Work out the finished part from the listing and answer in its coordinate system (mm). A direction names the side the tool comes from. Round coordinates to 2 decimals unless told otherwise and drop trailing zeros. Loops run counter-clockwise (first coordinate to the right, second up) from the corner with the lowest first, then second, coordinate; pieces in that order, holes last. Notation, with made-up numbers: (-21.5, 60) - (28.5, 60) arc R23 cw to (28.5, 94) - close; hole circle Ø3 at (-6.5, 85.25). An arc over 180 degrees is marked (long way). Return JSON: item names as keys, results as strings.
from build123d import *

# Parameters (mm, degrees)
F1_W     = 10
F1_H     = 10
F2_DEPTH = 1
F3_W     = 10
F3_H     = 1
F4_DEPTH = 12
F8_W     = 1
F8_H     = 15
F10_R    = 3


with BuildPart() as f2:
    # F1 (on Top) → F2 (new body)
    with BuildSketch(Plane.XY):
        with Locations((-1.3497796124, 5)):
            Rectangle(F1_W, F1_H)
    extrude(amount=F2_DEPTH)

    # F3 (on face) → F4 (join)
    with BuildSketch(Plane.XY.offset(1)):
        with Locations((-1.3497796124, 9.5)):
            Rectangle(F3_W, F3_H)
    extrude(amount=F4_DEPTH)

    # F8 (on 3pt) → F9 (join, up to the next surface of F2)
    with BuildSketch(Plane(origin=(0, -0.48, 0.36), x_dir=(-1, 0, 0), z_dir=(0, 0.8, -0.6))):
        with Locations((1.3497796124, 8.3)):
            Rectangle(F8_W, F8_H)
    extrude(until=Until.NEXT)

    # F10
    f10_edges = [f2.edges().sort_by_distance(p)[0] for p in [
        (3.65022, 0, 0.5),
        (-6.34978, 0, 0.5),
    ]]
    fillet(f10_edges, radius=F10_R)


solid = f2.part
1) A tool of negligible diameter and unlimited length cuts with its end or side. For faces 1 (the flat face through (-6.35, 9.3, 5)), 2 (the flat face through (1, 5, 1)), 3 (the flat face through (-4, 5, 1)), from which of +Z, -Z, +X, -X, +Y, -Y can it reach the whole face along a straight path? Write none if from no direction.
Verdict:
{"face 1": "+Z, -Z, -X, +Y, -Y", "face 2": "+Z, +X, -Y", "face 3": "+Z, -X, -Y"}
2) Find the intervals of material crossed by L1, parallel to Z at x = -3.25, y = 7; L2, parallel to X at y = 6.25, z = 9; L3, parallel to Y at x = -2, z = 4, in increasing order.
Verdict:
{"L1": "z = 0 to 1", "L2": "x = -1.85 to -0.85", "L3": "y = 9 to 10"}
3) Section B-B (x = -1.5) is taken. Give the vertices of the cut face in (y, z).
Verdict:
{"outline": "(0, 0) - (10, 0) - (10, 13) - (9, 13) - (0, 1) - close"}
4) Section D-D (x = 0) is taken. Give the vertices of the cut face in (y, z), and give its area (3 significant figures).
Verdict:
{"outline": "(0, 0) - (10, 0) - (10, 13) - (9, 13) - (9, 1) - (0, 1) - close", "area": "22.0 mm2"}
5) Flat-ended cylindrical pins translate along their axes: pin 1 (1.3 mm diameter, centred on x = -4.5, z = 6, fed in from -Y); pin 2 (2.5 mm diameter, centred on x = 2, y = 3.5, fed in from +Z); pin 3 (2 mm diameter, centred on y = 2, z = 1.5, fed in from +X). Find the tip coordinate at first contact, or state that the pin passes through.
Verdict:
{"pin 1": "stops at y = 9", "pin 2": "stops at z = 1", "pin 3": "stops at x = 3.65"}
6) Section A-A (z = 9) is taken. Give the vertices of the cut face in (x, y), and give its area (3 significant figures).
Verdict:
{"outline": "(-6.35, 9) - (-1.85, 9) - (-1.85, 6) - (-0.85, 6) - (-0.85, 9) - (3.65, 9) - (3.65, 10) - (-6.35, 10) - close", "area": "13.0 mm2"}
7) Section C-C (y = 5.25) is taken. Give the vertices of the cut face in (x, z), and give its area (3 significant figures).
Verdict:
{"outline": "(-6.35, 0) - (3.65, 0) - (3.65, 1) - (-0.85, 1) - (-0.85, 8) - (-1.85, 8) - (-1.85, 1) - (-6.35, 1) - close", "area": "17.0 mm2"}
